Part model, mm, in its own coordinate system. Face numbers are marked on the shaded views. A direction names the side the tool comes from. Round coordinates to 2 decimals unless told otherwise and drop trailing zeros. Write each loop counter-clockwise with the first axis right and the second up, starting at its lowest first coordinate (ties: lowest second). Pieces come first, ordered by that corner, then holes. Notation, with made-up numbers: (-8.5, 49.5) -> (43.5, 49.5) arc R31 ccw to (43.5, 79.5) -> close; hole circle Ø7 at (15.5, 18). An arc over 180 degrees is marked (long way). Return JSON: item names as keys, results as strings. Group by question number.
```python
from build123d import *

# Parameters (mm, degrees)
SKETCH1_W                      = 64.77
SKETCH1_H                      = 50.8
SKETCH1_R                      = 2.5527
SKETCH1_R_2                    = 7.9375
BOSS_EXTRUDE1_DEPTH            = 12.7
F_7_0_201_DIAMETER_HOLE1_D     = 5.1054
F_7_0_201_DIAMETER_HOLE1_DEPTH = 70.104
F_7_0_201_DIAMETER_HOLE1_TIP   = 1.533816902
SKETCH6_R                      = 3.9624
CUT_EXTRUDE1_DEPTH             = 4.826
SKETCH7_W                      = 20.32
SKETCH7_H                      = 25.4
CUT_EXTRUDE2_DEPTH             = 49.543247728
FILLET2_R                      = 9.525


with BuildPart() as part:
    # Sketch1 → Boss-Extrude1 (new body)
    with BuildSketch(Plane.XY):
        with Locations((6.985, 0)):
            Rectangle(SKETCH1_W, SKETCH1_H)
        with Locations(Location((-19.05, 19.05, 0), (0, 0, 180))):
            Circle(SKETCH1_R, mode=Mode.SUBTRACT)
        with Locations((19.05, 19.05)):
            Circle(SKETCH1_R, mode=Mode.SUBTRACT)
        with Locations((19.05, -19.05)):
            Circle(SKETCH1_R, mode=Mode.SUBTRACT)
        with Locations((10.16, -19.05)):
            Circle(SKETCH1_R, mode=Mode.SUBTRACT)
        with Locations((14.605, 0)):
            Circle(SKETCH1_R_2, mode=Mode.SUBTRACT)
    extrude(amount=BOSS_EXTRUDE1_DEPTH)

    # #7 (0.201) Diameter Hole1
    with Locations(Plane(origin=(-24.721209515, -12.864288698, 0), x_dir=(1, 0, 0), z_dir=(0, 0, -1))):
        with Locations((57.741209515, 6.185711302), (57.741209515, -31.914288698), (43.771209515, -24.294288698)):
            Hole(F_7_0_201_DIAMETER_HOLE1_D / 2, depth=F_7_0_201_DIAMETER_HOLE1_DEPTH)
            with Locations((0, 0, -(F_7_0_201_DIAMETER_HOLE1_DEPTH + F_7_0_201_DIAMETER_HOLE1_TIP / 2))):  # 118° drill point
                Cone(0, F_7_0_201_DIAMETER_HOLE1_D / 2, F_7_0_201_DIAMETER_HOLE1_TIP, mode=Mode.SUBTRACT)

    # Sketch6 → Cut-Extrude1 (cut)
    with BuildSketch(Plane(origin=(0, 0, 12.7), x_dir=(-1, 0, 0), z_dir=(0, 0, -1))):
        with Locations((-19.05, 19.05)):
            Circle(SKETCH6_R)
        with Locations((-19.05, -19.05)):
            Circle(SKETCH6_R)
        with Locations((-10.16, -19.05)):
            Circle(SKETCH6_R)
        with Locations((19.05, 19.05)):
            Circle(SKETCH6_R)
    extrude(amount=CUT_EXTRUDE1_DEPTH, mode=Mode.SUBTRACT)

    # Sketch7 → Cut-Extrude2 (cut, through all)
    with BuildSketch(Plane(origin=(0, 0, 0), x_dir=(-1, 0, 0), z_dir=(0, 0, -1))):
        with Locations((15.24, -12.7)):
            Rectangle(SKETCH7_W, SKETCH7_H)
    extrude(amount=-CUT_EXTRUDE2_DEPTH, mode=Mode.SUBTRACT)

    # Fillet2
    fillet2_edges = [part.edges().sort_by_distance(p)[0] for p in [
        (-5.08, 0, 6.35),
    ]]
    fillet(fillet2_edges, radius=FILLET2_R)


solid = part.part
```
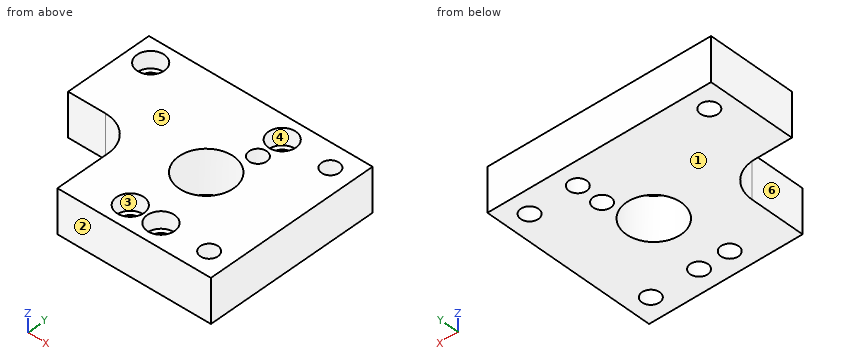
Item 1: Which spindle directions (+Z, -Z, +X, -X, +Y, -Y) get a long thin tool onto all of the face, cutting with end or side? Do the marked faces 4, 5 and 6. Say none if no direction does.
Item 2: Cut at A-A (y = 19.05). Write the cut outline in (x, z), then the cut area to 3 significant figures.
Item 3: Flat gauge pins, fed straight in: P1, Ø3, axis at x = -22.5, z = 8, coming from the -Y side; P2, Ø1.5, axis at y = -14.5, z = 8.5, coming from the -X side; P3, Ø4.5, axis at x = 33.02, y = 19.05, coming from the -Z side; P4, Ø7, axis at x = -19.05, y = 19.05, coming from the +Z side. Where does each tip first touch, or does it go through?
Item 4: Cut at B-B (x = -19.05). Write the cut outline in (y, z), then the cut area to 3 significant figures.
Item 5: Wall check: L1, parallel to Y at x = 33.02, z = 9; L2, parallel to Y at x = -19.05, z = 4; L3, parallel to Y at x = -19, z = 10. Give the ranges that are in metal, low to high.
Item 6: Cut at D-D (x = 33.02). Write the cut outline in (y, z), then the cut area to 3 significant figures.
Item 7: Cut at C-C (z = 9.75). State how many separate pieces and enclosed holes the cut face has, then the cut area to 3 significant figures.
Item 8: Two-plate mould, pull along Y, no slides. Class the marked faces 1, 2 and 3: released by +Y, released by -Y, zero draft, split by the parting line, or undercut.
Checks:
{
 "1": {"face 4": "+Z", "face 5": "+Z, +X, -X, +Y, -Y", "face 6": "+Z, -Z, -X, -Y"},
 "2": {"outline": "(-25.4, 0) -> (-21.6, 0) -> (-21.6, 7.87) -> (-23.01, 7.87) -> (-23.01, 12.7) -> (-25.4, 12.7) -> close; (-16.5, 0) -> (16.5, 0) -> (16.5, 7.87) -> (15.09, 7.87) -> (15.09, 12.7) -> (-15.09, 12.7) -> (-15.09, 7.87) -> (-16.5, 7.87) -> close; (21.6, 0) -> (30.47, 0) -> (30.47, 12.7) -> (23.01, 12.7) -> (23.01, 7.87) -> (21.6, 7.87) -> close; (35.57, 0) -> (39.37, 0) -> (39.37, 12.7) -> (35.57, 12.7) -> close", "area": "601 mm2"},
 "3": {"P1": "stops at y = 0", "P2": "stops at x = -5.08", "P3": "passes through", "P4": "stops at z = 7.87"},
 "4": {"outline": "(0, 0) -> (16.5, 0) -> (16.5, 7.87) -> (15.09, 7.87) -> (15.09, 12.7) -> (0, 12.7) -> close; (21.6, 0) -> (25.4, 0) -> (25.4, 12.7) -> (23.01, 12.7) -> (23.01, 7.87) -> (21.6, 7.87) -> close", "area": "244 mm2"},
 "5": {"L1": "y = -25.4 to -21.6, -16.5 to 16.5, 21.6 to 25.4", "L2": "y = 0 to 16.5, 21.6 to 25.4", "L3": "y = 0 to 15.09, 23.01 to 25.4"},
 "6": {"outline": "(-25.4, 0) -> (-21.6, 0) -> (-21.6, 12.7) -> (-25.4, 12.7) -> close; (-16.5, 0) -> (16.5, 0) -> (16.5, 12.7) -> (-16.5, 12.7) -> close; (21.6, 0) -> (25.4, 0) -> (25.4, 12.7) -> (21.6, 12.7) -> close", "area": "515 mm2"},
 "7": {"separate pieces": "1", "enclosed holes": "8", "area": "2,340 mm2"},
 "8": {"face 1": "zero draft", "face 2": "released by -Y", "face 3": "undercut"}
}
